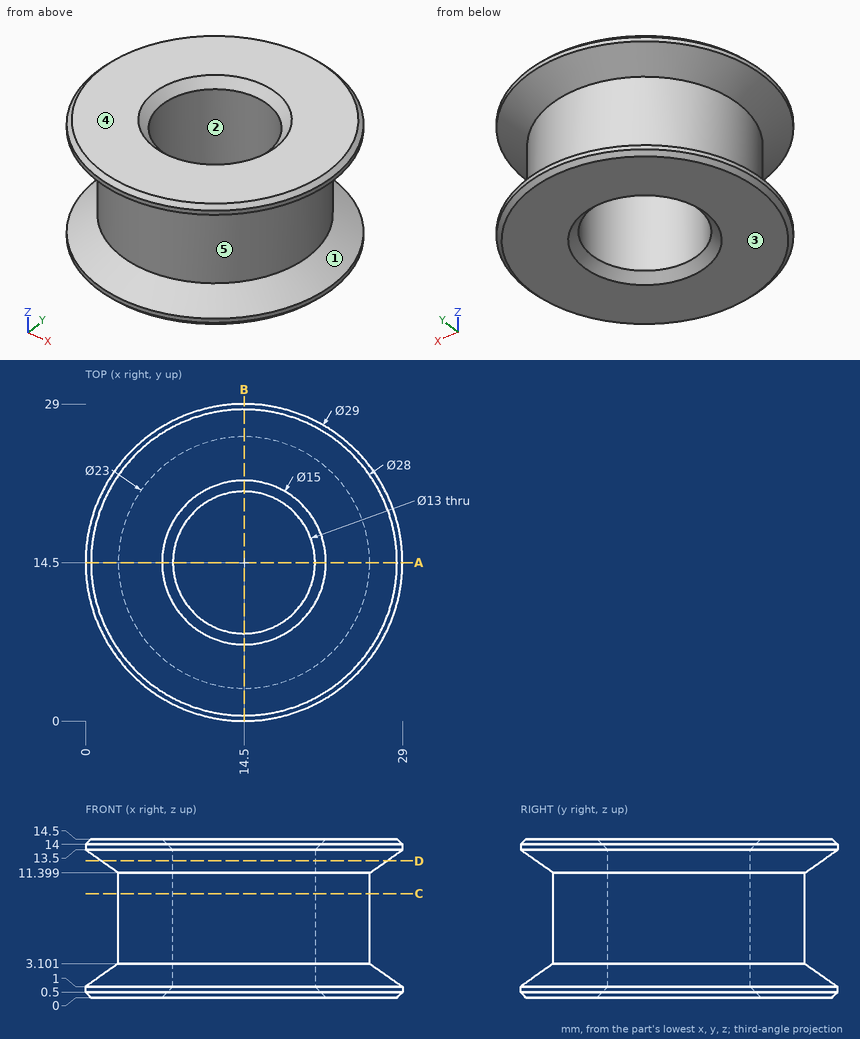
Could you check a few things on this drawing? It's one solid part, dimensions in mm from its lowest x, y, z. A direction names the side the tool comes from. Round coordinates to 2 decimals unless told otherwise and drop trailing zeros. Write each loop counter-clockwise with the first axis right and the second up, starting at its lowest first coordinate (ties: lowest second). Pieces come first, ordered by that corner, then holes. Notation, with made-up numbers: (83.25, -10) -> (136.25, -10) arc R32 cw to (136.25, 26) -> close; hole circle Ø11 at (24, 6). An arc over 180 degrees is marked (long way). Use one line per item in the form item = value. Start each with the question number.
Q1. We'd pull the mould along X, two halves only. Please class the marked faces 1, 2 and 3: +X half, -X half, draft (parallel to the pull), parting line (faces both ways), or undercut.
Q2. Imagine slicing it at A-A (y = 14.5). Please give me the cut outline in (x, z), then the cut area to 3 significant figures.
Q3. If I drill on probe 1 along Y at (x, z) = (14.5, 9.75); probe 2 along X at (y, z) = (11.75, 2.75); probe 3 along Y at (x, z) = (17, 7.25) (1 decimal), over which ranges is the centre line in solid material (lowest first)? Write a range as [from, to].
Q4. Imagine slicing it at C-C (z = 9.5). Please give me the cut outline in (x, y).
Q5. Imagine slicing it at D-D (z = 12.5). Please give me the cut outline in (x, y), then the cut area to 3 significant figures.
Q6. Which directions (+Z, -Z, +X, -X, +Y, -Y) give clear straight access to the entire face, cutting with the end or side of a thin tool? Please do the marked faces 4 and 5.
Q7. I'm going to push flat-ended pins straight in: P1, Ø8, axis at y = 22.5, z = 10, coming from the -X side; P2, Ø8, axis at y = 7, z = 2, coming from the +X side; P3, Ø1.5, axis at x = 17.5, z = 11, coming from the -Y side (1 decimal). Where does each tip first touch, or does it pass through?
Worked out:
q1.face_1 = parting line
q1.face_2 = undercut
q1.face_3 = draft
q2.outline = (0, 0.5) -> (0.5, 0) -> (7, 0) -> (8, 1) -> (8, 13.5) -> (7, 14.5) -> (0.5, 14.5) -> (0, 14) -> (0, 13.5) -> (3, 11.4) -> (3, 3.1) -> (0, 1) -> close; (21, 1) -> (22, 0) -> (28.5, 0) -> (29, 0.5) -> (29, 1) -> (26, 3.1) -> (26, 11.4) -> (29, 13.5) -> (29, 14) -> (28.5, 14.5) -> (22, 14.5) -> (21, 13.5) -> close
q2.area = 167 mm^2
q3.probe_1 = [3, 8], [21, 26]
q3.probe_2 = [2.82, 8.61], [20.39, 26.18]
q3.probe_3 = [3.3, 8.5], [20.5, 25.7]
q4.outline = circle Ø23 at (14.5, 14.5); hole circle Ø13 at (14.5, 14.5)
q5.outline = circle Ø26.14 at (14.5, 14.5); hole circle Ø13 at (14.5, 14.5)
q5.area = 404 mm^2
q6.face_4 = +Z, +X, -X, +Y, -Y
q6.face_5 = none
q7.P1 = 1.33
q7.P2 = 28.54
q7.P3 = 2.9
